Part model, mm, in its own coordinate system. A direction names the side the tool comes from. Give positions to 0.01 mm unless a question says otherwise; leave off trailing zeros. Order: outer loops, then holes, each group sorted by start corner. A loop starts at its lowest first (then second) coordinate and runs counter-clockwise, first axis right, second up. Notation, with made-up numbers: M 11.5,-18.75 L 20.5,-18.75 A23 ccw 20.5,6.25 Z; hole C 34.5,51.5 d8. An arc over 180 degrees is marked long. Return JSON: item names as keys, results as strings.
from build123d import *

# Parameters (mm, degrees)
F0_W     = 374.65
F0_H     = 254
F1_DEPTH = 19.05
F3_DEPTH = 152.4
F5_DEPTH = 203.2


with BuildPart() as f1:
    # F0 (on Top) → F1 (new body)
    with BuildSketch(Plane.XY):
        Rectangle(F0_W, F0_H)
        with BuildLine():
            Line((47.498, 9.398), (142.748, 9.398))
            ThreePointArc((142.748, 9.398), (144.9930640303, 8.4680640303), (145.923, 6.223))
            Line((145.923, 6.223), (145.923, -22.479))
            ThreePointArc((145.923, -22.479), (144.9930640303, -24.7240640303), (142.748, -25.654))
            Line((142.748, -25.654), (47.498, -25.654))
            ThreePointArc((47.498, -25.654), (45.2529359697, -24.7240640303), (44.323, -22.479))
            Line((44.323, -22.479), (44.323, 6.223))
            ThreePointArc((44.323, 6.223), (45.2529359697, 8.4680640303), (47.498, 9.398))
        make_face(mode=Mode.SUBTRACT)
    extrude(amount=-F1_DEPTH)

    # F2 (on Front) → F3 (cut, symmetric)
    with BuildSketch(Plane.XZ):
        with BuildLine():
            Line((187.325, 0), (179.3748, 0))
            Line((179.3748, 0), (179.3748, -1.6002))
            ThreePointArc((179.3748, -1.6002), (183.8649280605, -3.4600719395), (185.7248, -7.9502))
            Line((185.7248, -7.9502), (187.325, -7.9502))
            Line((187.325, -7.9502), (187.325, 0))
        make_face()
        with BuildLine():
            Line((-179.3748, -1.6002), (-179.3748, 0))
            Line((-179.3748, 0), (-187.325, 0))
            Line((-187.325, 0), (-187.325, -7.9502))
            Line((-187.325, -7.9502), (-185.7248, -7.9502))
            ThreePointArc((-185.7248, -7.9502), (-183.8649280605, -3.4600719395), (-179.3748, -1.6002))
        make_face()
    extrude(amount=F3_DEPTH, both=True, mode=Mode.SUBTRACT)

    # F4 (on Right) → F5 (cut, symmetric)
    with BuildSketch(Plane.YZ):
        with BuildLine():
            Line((127, 0), (119.0498, 0))
            Line((119.0498, 0), (119.0498, -1.6002))
            ThreePointArc((119.0498, -1.6002), (123.5399280605, -3.4600719395), (125.3998, -7.9502))
            Line((125.3998, -7.9502), (127, -7.9502))
            Line((127, -7.9502), (127, 0))
        make_face()
        with BuildLine():
            Line((-119.0498, -1.6002), (-119.0498, 0))
            Line((-119.0498, 0), (-127, 0))
            Line((-127, 0), (-127, -7.9502))
            Line((-127, -7.9502), (-125.3998, -7.9502))
            ThreePointArc((-125.3998, -7.9502), (-123.5399280605, -3.4600719395), (-119.0498, -1.6002))
        make_face()
    extrude(amount=F5_DEPTH, both=True, mode=Mode.SUBTRACT)


solid = f1.part
Q1. Band-saw the part on B-B (y = -10). Give the cut face in (x, z) (3 decimals), then the cut area to 3 significant figures.
Established:
{"outline": "M -187.325,-19.05 L 44.323,-19.05 L 44.323,0 L -179.375,0 L -179.375,-1.6 A6.35 ccw -185.725,-7.95 L -187.325,-7.95 Z; M 145.923,-19.05 L 187.325,-19.05 L 187.325,-7.95 L 185.725,-7.95 A6.35 ccw 179.375,-1.6 L 179.375,0 L 145.923,0 Z", "area": "5,140 mm²"}
Q2. Band-saw the part on A-A (x = 66.5). Give the cut face in (y, z).
Established:
{"outline": "M -127,-19.05 L -25.65,-19.05 L -25.65,0 L -119.05,0 L -119.05,-1.6 A6.35 ccw -125.4,-7.95 L -127,-7.95 Z; M 9.4,-19.05 L 127,-19.05 L 127,-7.95 L 125.4,-7.95 A6.35 ccw 119.05,-1.6 L 119.05,0 L 9.4,0 Z"}
Q3. Band-saw the part on C-C (z = -13.5). Give the cut face in (x, y) (3 decimals), then the cut area to 3 significant figures.
Established:
{"outline": "M -187.325,-127 L 187.325,-127 L 187.325,127 L -187.325,127 Z; hole M 44.323,-22.479 A3.175 ccw 47.498,-25.654 L 142.748,-25.654 A3.175 ccw 145.923,-22.479 L 145.923,6.223 A3.175 ccw 142.748,9.398 L 47.498,9.398 A3.175 ccw 44.323,6.223 Z", "area": "91,600 mm²"}
Q4. 3-axis set-ups, long thin cutter, end or side, ignore diameter. For faces 1 (the flat face through (145.923, -8, -9)), 2 (the flat face through (-3, -127, -13)): which of +Z, -Z, +X, -X, +Y, -Y reach the whole face in a straight line?
Established:
{"face 1": "+Z, -Z", "face 2": "+Z, -Z, +X, -X, -Y"}
Q5. Pin check, flat tips, straight feed: pin 1 (3 mm diameter, centred on y = -70.5, z = -4, fed in from -X); pin 2 (10 mm diameter, centred on x = -39, z = -3.5, fed in from +Y); pin 3 (0.5 mm diameter, centred on y = 41.5, z = -1, fed in from -X); pin 4 (0.5 mm diameter, centred on x = -24, z = -0.5, fed in from +Y). Stop position of each tip, or through.
Established:
{"pin 1": "stops at x = -185.23", "pin 2": "stops at y = 127", "pin 3": "stops at x = -179.37", "pin 4": "stops at y = 119.05"}
Q6. Two-plate mould, pull along Y, no slides. Class faces 3 (the flat face through (-3, 127, -13)), 4 (the flat face through (-3, 2, 0)), 5 (the flat face through (94, 9.398, -9)): +Y half, -Y half, draft (parallel to the pull), parting line (faces both ways), or undercut.
Established:
{"face 3": "+Y half", "face 4": "draft", "face 5": "undercut"}
Q7. Probe line 1 along Y through (x, z) = (135, -0.75); line 2 along Y through (x, z) = (108.5, -12.25); line 3 along Y through (x, z) = (-47, -1.5). List the from-to ranges inside material, lowest first.
Established:
{"line 1": "y = -119.05 to -25.65, 9.4 to 119.05", "line 2": "y = -127 to -25.65, 9.4 to 127", "line 3": "y = -119.05 to 119.05"}
